Can you work these out from the drawing? Everything is in mm from the part's minimum corner. Coordinates: 2 decimals unless noted, no trailing zeros. Loops run counter-clockwise (first coordinate to the right, second up) from the corner with the lowest first, then second, coordinate; pieces in that order, holes last. Notation, with made-up numbers: (1.25, 64.5) - (20.25, 64.5) arc R18 cw to (20.25, 96.5) - close; hole circle Ø10 at (5.5, -8.5). An arc over 180 degrees is marked (long way). One line per question, with ' | ' between items. Start each with the question number.
1. I'm going to push flat-ended pins straight in: P1, Ø4.5, axis at x = 10, y = 10, coming from the -Z side; P2, Ø10, axis at x = 38, z = 2.5, coming from the -Y side; P3, Ø5, axis at x = 199.5, y = 5, coming from the +Z side; P4, Ø4.5, axis at x = 134, z = 11, coming from the -Y side. Where does each tip first touch, or does it pass through?
2. I want a section at B-B, the plane y = 5. Write out the boundary of the cut face in (x, z), then the cut area to 3 significant figures.
3. Please list where these lines run through material, in increasing order: L1, parallel to X at y = 11.75, z = 2.25; L2, parallel to Z at x = 106, y = 16; L3, parallel to Y at x = 30, z = 2. Write a range as [from, to].
4. I want a section at D-D, the plane z = 15. Write out the boundary of the cut face in (x, y), then the cut area to 3 significant figures.
5. I want a section at C-C, the plane x = 176.5. Write out the boundary of the cut face in (y, z), then the cut area to 3 significant figures.
6. I want a section at A-A, the plane x = 10. Write out the boundary of the cut face in (y, z).
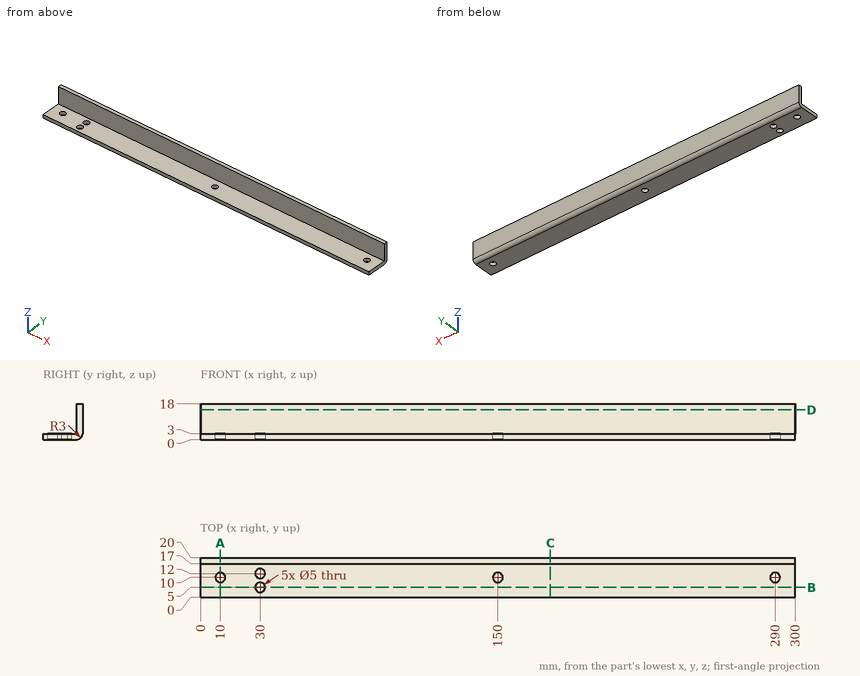
Results are:
1) P1: passes through | P2: stops at y = 0 | P3: stops at z = 3 | P4: stops at y = 17
2) outline: (0, 0) - (27.5, 0) - (27.5, 3) - (0, 3) - close; (32.5, 0) - (300, 0) - (300, 3) - (32.5, 3) - close | area: 885 mm2
3) L1: x = [0, 8.21], [11.79, 27.51], [32.49, 148.21], [151.79, 288.21], [291.79, 300] | L2: z = [0, 3] | L3: y = [0, 2.5], [7.5, 9.5], [14.5, 19.83]
4) outline: (0, 17) - (300, 17) - (300, 20) - (0, 20) - close | area: 900 mm2
5) outline: (0, 0) - (17, 0) arc R3 ccw to (20, 3) - (20, 18) - (17, 18) - (17, 3) - (0, 3) - close | area: 103 mm2
6) outline: (0, 0) - (7.5, 0) - (7.5, 3) - (0, 3) - close; (12.5, 0) - (17, 0) arc R3 ccw to (20, 3) - (20, 18) - (17, 18) - (17, 3) - (12.5, 3) - close
